Geometry: see drawing. Coordinates: mm, zero at the bounding-box minimum. Round coordinates to 2 decimals unless told otherwise and drop trailing zeros. Write each loop counter-clockwise with the first axis right and the second up, starting at its lowest first coordinate (ties: lowest second). Pieces come first, ordered by that corner, then holes.
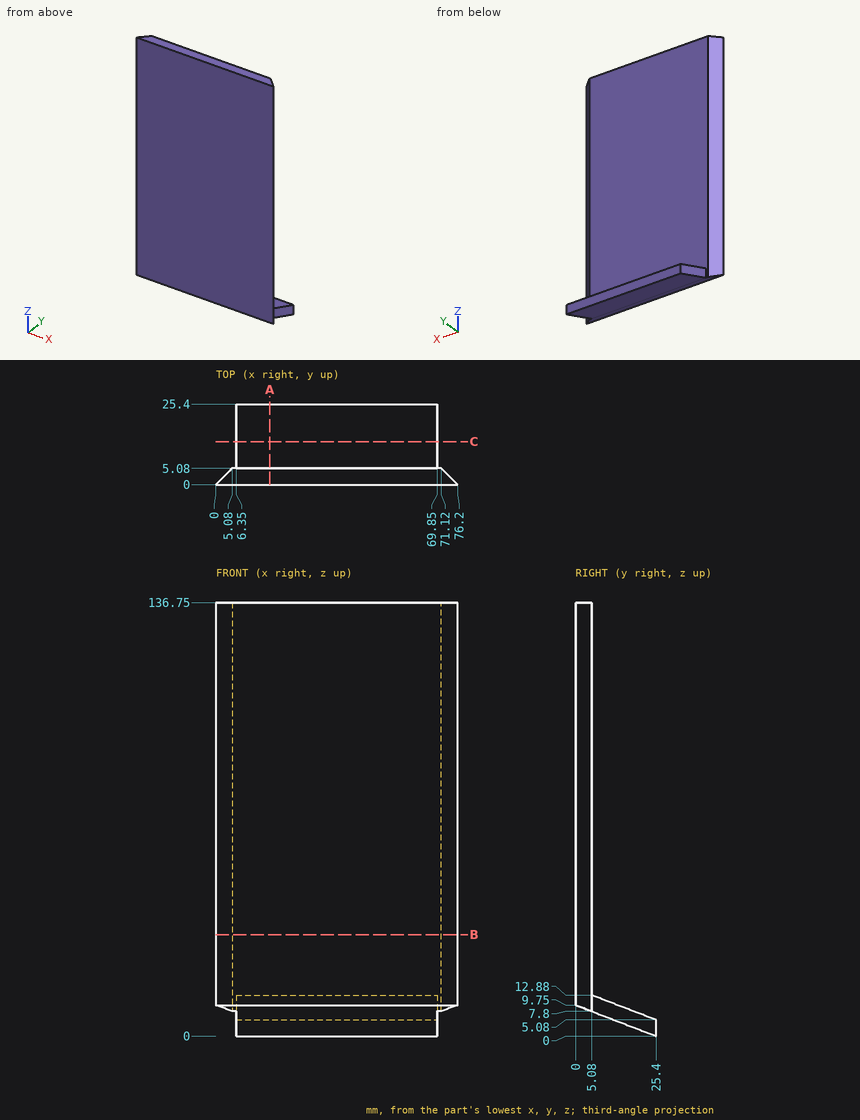
Q1. Line query: line 1 (Y direction, x = 69.5, z = 123.5); line 2 (Z direction, x = 45, y = 16.75); line 3 (Z direction, x = 13, y = 4.5). Output: solid intervals per line, ascending.
Q2. Section query C-C, the plane y = 13.5. Output: boundary loops of the cut face in (x, z).
Q3. Pin query (flat end, axial travel): P1, Ø4, axis at y = 18.5, z = 9, coming from the +X side; P2, Ø1.5, axis at x = 25, y = 5.5, coming from the -Z side; P3, Ø1, axis at y = 4.5, z = 83.5, coming from the +X side. Return the tip coordinate at first contact, or that it passes through.
Q4. Section query A-A, the plane x = 17. Output: boundary loops of the cut face in (y, z), and give its area (3 significant figures).
Q5. Section query B-B, the plane z = 32. Output: boundary loops of the cut face in (x, y), and give its area (3 significant figures).
Filled in:
1. line 1: y = 0 to 5.08
1. line 2: z = 3.32 to 8.4
1. line 3: z = 8.02 to 136.75
2. outline: (6.35, 4.57) - (69.85, 4.57) - (69.85, 9.65) - (6.35, 9.65) - close
3. P1: stops at x = 69.85
3. P2: stops at z = 7.35
3. P3: stops at x = 72.2
4. outline: (0, 9.75) - (25.4, 0) - (25.4, 5.08) - (5.08, 12.88) - (5.08, 136.75) - (0, 136.75) - close
4. area: 753 mm2
5. outline: (0, 0) - (76.2, 0) - (71.12, 5.08) - (5.08, 5.08) - close
5. area: 361 mm2
